Input: part model. Units: mm. Frame: model coordinates. Face numbers are marked on the shaded views. Coordinates: 2 decimals unless noted, no trailing zeros. Loops run counter-clockwise (first coordinate to the right, second up) from the corner with the lowest first, then second, coordinate; pieces in that order, holes last. Notation, with made-up numbers: (42, -39) - (48, -39) arc R24 ccw to (48, -29) - close; hole circle Ø2 at (-27.75, 77). An arc over 180 degrees is marked (long way). Use a Markdown table: item, result. Add a question column.
1. Draft query along Z for the marked faces 1, 2 and 3. Return one class per face: released by +Z, released by -Z, zero draft, split by the parting line, or undercut.
2. Section query A-A on y = 0. Return the cut outline in (x, z) (3 decimals), then the cut area to 3 significant figures.
3. Ray query, L1, parallel to Z at x = 18.5, y = 0 (3 decimals); L2, parallel to Z at x = 26, y = 0 (3 decimals); L3, parallel to Y at x = 32, z = -17.5. Return the intervals inside material, ascending. Write a range as [from, to].
4. Contact query for flat-ended pins moving along their axis: P1, Ø5, axis at x = 15, y = -13.5, coming from the +Z side; P2, Ø6, axis at x = 13, z = 26, coming from the +Y side; P3, Ø1, axis at x = 20.5, y = 29, coming from the +Z side. Output: stop coordinate, or through.
5. Section query B-B on z = 0. Return the cut outline in (x, y) (3 decimals).
6. Section query D-D on y = -22.5. Return the cut outline in (x, z).
```python
from build123d import *

# Parameters (mm, degrees)
F0_R            = 38.1
F1_DEPTH        = 38.1
F3_START        = 19.05
F2_W            = 12.7
F2_H            = 3.175
F3_DEPTH        = 19.05
F3_COPIES_COUNT = 5
F4_R            = 9.525
F5_DEPTH        = 38.101


# Not quite as in the source:
# - a pattern or mirror of a feature is missing from the dataset's text; its kind, count and spacing are read off the source's solid


with BuildPart() as f1:
    # F0 (on Right) → F1 (new body)
    with BuildSketch(Plane.YZ):
        Circle(F0_R)
    extrude(amount=F1_DEPTH)

    # F2 (on Top) → F3 (cut)
    with BuildSketch(Plane.XY.offset(F3_START)):
        with Locations((31.75, 0)):
            Rectangle(F2_W, F2_H)
    f3 = extrude(amount=F3_DEPTH, mode=Mode.SUBTRACT)

    # F3_copies: F3 ×5 about axis
    f3_copies_axis = Axis((0, 0, 0), (1, 0, 0))
    for i in range(1, F3_COPIES_COUNT):
        add(f3.rotate(f3_copies_axis, i * 360 / F3_COPIES_COUNT), mode=Mode.SUBTRACT)

    # F4 (on face) → F5 (cut, through all)
    with BuildSketch(Plane.YZ.offset(38.1)):
        Circle(F4_R)
    extrude(amount=-F5_DEPTH, mode=Mode.SUBTRACT)


solid = f1.part
```
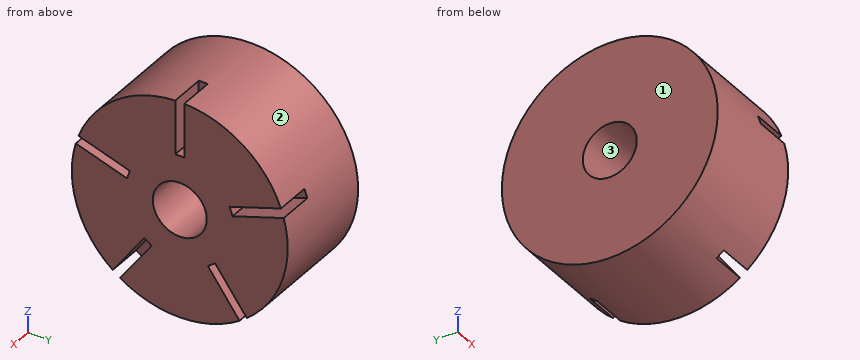
Resolved:
| question | item | result |
|---|---|---|
| 1 | face 1 | zero draft |
| 1 | face 2 | split by the parting line |
| 1 | face 3 | undercut |
| 2 | outline | (0, -38.1) - (38.1, -38.1) - (38.1, -9.525) - (0, -9.525) - close; (0, 9.525) - (38.1, 9.525) - (38.1, 19.05) - (25.4, 19.05) - (25.4, 38.1) - (0, 38.1) - close |
| 2 | area | 1,940 mm² |
| 3 | L1 | [-38.1, -9.525], [9.525, 38.1] |
| 3 | L2 | [-38.1, -9.525], [9.525, 19.05] |
| 3 | L3 | [-33.84, -14.68], [-10.75, 10.75], [14.68, 33.84] |
| 4 | P1 | z = 36.48 |
| 4 | P2 | y = 30.37 |
| 4 | P3 | z = 25.29 |
| 5 | outline | (0, -38.1) - (38.1, -38.1) - (38.1, -9.525) - (0, -9.525) - close; (0, 9.525) - (38.1, 9.525) - (38.1, 38.1) - (0, 38.1) - close |
| 6 | outline | (0, -30.75) - (25.4, -30.75) - (25.4, -28.27) - (38.1, -28.27) - (38.1, 5.64) - (25.4, 5.64) - (25.4, 8.98) - (38.1, 8.98) - (38.1, 30.75) - (0, 30.75) - close |
